```python
from build123d import *

# Parameters (mm, degrees)
EXTRUDE_START          = -12.5
EXTRUDE_1_DEPTH        = 25
EXTRUDE_ROTATE_1_ANGLE = 8
EXTRUDE_START_2        = -8.5
EXTRUDE_SKETCH_2_W     = 410
EXTRUDE_SKETCH_2_H     = 310
EXTRUDE_2_DEPTH        = 3
EXTRUDE_ROTATE_2_ANGLE = 8
EXTRUDE_START_3        = -30.5
EXTRUDE_SKETCH_3_W     = 80
EXTRUDE_SKETCH_3_H     = 80
EXTRUDE_3_DEPTH        = 22
EXTRUDE_ROTATE_3_ANGLE = 8


with BuildPart() as part:
    # Extrude sketch 1 → Extrude 1 (new body)
    with BuildSketch(Plane.XY.offset(EXTRUDE_START)):
        with BuildLine():
            Line((219, 175), (-219, 175))
            ThreePointArc((-219, 175), (-223.242640687, 173.242640687), (-225, 169))
            Line((-225, 169), (-225, -169))
            ThreePointArc((-225, -169), (-223.242640687, -173.242640687), (-219, -175))
            Line((-219, -175), (219, -175))
            ThreePointArc((219, -175), (223.242640687, -173.242640687), (225, -169))
            Line((225, -169), (225, 169))
            ThreePointArc((225, 169), (223.242640687, 173.242640687), (219, 175))
        make_face()
        with BuildLine():
            Line((203, 155), (-203, 155))
            ThreePointArc((-203, 155), (-204.414213562, 154.414213562), (-205, 153))
            Line((-205, 153), (-205, -153))
            ThreePointArc((-205, -153), (-204.414213562, -154.414213562), (-203, -155))
            Line((-203, -155), (203, -155))
            ThreePointArc((203, -155), (204.414213562, -154.414213562), (205, -153))
            Line((205, -153), (205, 153))
            ThreePointArc((205, 153), (204.414213562, 154.414213562), (203, 155))
        make_face(mode=Mode.SUBTRACT)
    extrude(amount=EXTRUDE_1_DEPTH)


with BuildPart() as part_1:
    # Extrude rotate 1: moved
    add(part.part.rotate(Axis((0, 0, 0), (0, 1, 0)), EXTRUDE_ROTATE_1_ANGLE))


with BuildPart() as part_2:
    # Extrude place 1: moved
    add(part_1.part.moved(Location((588.929348295, 0, 623.692298575))))


with BuildPart() as body_2:
    # Extrude sketch 2 → Extrude 2 (new body)
    with BuildSketch(Plane.XY.offset(EXTRUDE_START_2)):
        Rectangle(EXTRUDE_SKETCH_2_W, EXTRUDE_SKETCH_2_H)
    extrude(amount=EXTRUDE_2_DEPTH)


with BuildPart() as body_2_1:
    # Extrude rotate 2: moved
    add(body_2.part.rotate(Axis((0, 0, 0), (0, 1, 0)), EXTRUDE_ROTATE_2_ANGLE))


with BuildPart() as body_2_2:
    # Extrude place 2: moved
    add(body_2_1.part.moved(Location((588.929348295, 0, 623.692298575))))


with BuildPart() as body_3:
    # Extrude sketch 3 → Extrude 3 (new body)
    with BuildSketch(Plane.XY.offset(EXTRUDE_START_3)):
        with Locations((100, 0)):
            Rectangle(EXTRUDE_SKETCH_3_W, EXTRUDE_SKETCH_3_H)
    extrude(amount=EXTRUDE_3_DEPTH)


with BuildPart() as body_3_1:
    # Extrude rotate 3: moved
    add(body_3.part.rotate(Axis((0, 0, 0), (0, 1, 0)), EXTRUDE_ROTATE_3_ANGLE))


with BuildPart() as body_3_2:
    # Extrude place 3: moved
    add(body_3_1.part.moved(Location((588.929348295, 0, 623.692298575))))


with BuildPart() as part_3:
    add(part_2.part)

    # Combine (weld / assembly of features): union body 3, body 2
    add(body_3_2.part)
    add(body_2_2.part)


solid = part_3.part
```
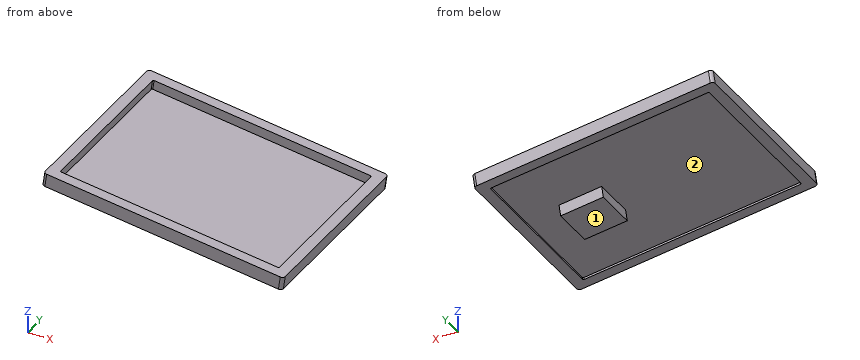
Part model, mm, in its own coordinate system. Face numbers are marked on the shaded views. Round coordinates to 2 decimals unless told otherwise and drop trailing zeros. Loops run counter-clockwise (first coordinate to the right, second up) from the corner with the lowest first, then second, coordinate; pieces in that order, holes last.
1. Slice it at C-C (x = 527). Give the cut face in (y, z).
Solutions:
outline: (-175, 619.77) - (-155, 619.77) - (-155, 623.81) - (155, 623.81) - (155, 619.77) - (175, 619.77) - (175, 645.02) - (155, 645.02) - (155, 626.84) - (-155, 626.84) - (-155, 645.02) - (-175, 645.02) - close
2. Slice it at A-A (y = 8). Give the cut face in (x, z), and give its area (3 significant figures).
Solutions:
outline: (364.38, 642.63) - (384.18, 639.84) - (384.74, 643.81) - (647.16, 606.92) - (644.1, 585.14) - (723.32, 574) - (726.38, 595.79) - (790.75, 586.74) - (790.19, 582.78) - (810, 580) - (813.48, 604.76) - (793.67, 607.54) - (791.17, 589.72) - (385.16, 646.78) - (387.66, 664.6) - (367.86, 667.38) - close
area: 3,990 mm2
3. Two-plate mould, pull along Y, no slides. Class the marked faces 1 and 2: pulls with the +Y half, pulls with the -Y half, needs draft (parallel to the pull), parting line crosses it, or undercut.
Solutions:
face 1: needs draft
face 2: undercut
4. Slice it at B-B (z = 623). Give the cut face in (x, y), and give its area (3 significant figures).
Solutions:
outline: (504.04, -175) - (683.67, -175) - (683.67, -155) - (554.34, -155) - (554.34, 155) - (683.67, 155) - (683.67, 175) - (504.04, 175) - (504.04, 155) - (532.78, 155) - (532.78, -155) - (504.04, -155) - close
area: 13,900 mm2
5. Slice it at D-D (x = 689). Give the cut face in (y, z), and give its area (3 significant figures).
Solutions:
outline: (-175, 597.01) - (-155, 597.01) - (-155, 601.04) - (-40, 601.04) - (-40, 578.83) - (40, 578.83) - (40, 601.04) - (155, 601.04) - (155, 597.01) - (175, 597.01) - (175, 622.25) - (155, 622.25) - (155, 604.07) - (-155, 604.07) - (-155, 622.25) - (-175, 622.25) - close
area: 3,730 mm2
6. Drill centre lines: line 1 along Y through (x, z) = (595, 621.5); line 2 along Z through (x, y) = (413, -25); line 3 along Z through (x, y) = (674.5, 103.5). Where is each one in solid material? Low to high.
Solutions:
line 1: y = -175 to -155, 155 to 175
line 2: z = 639.83 to 642.86
line 3: z = 603.08 to 606.11
7. Flat gauge pins, fed straight in: pin 1 (6 mm diameter, centred on x = 597, y = -23, fed in from +Z); pin 2 (16.5 mm diameter, centred on x = 672, z = 597, fed in from +Y); pin 3 (1.5 mm diameter, centred on x = 516, y = 99, fed in from -Z); pin 4 (5 mm diameter, centred on x = 532.5, y = 55, fed in from +Z). Where does each tip first touch, or does it go through?
Solutions:
pin 1: stops at z = 617.43
pin 2: stops at y = 175
pin 3: stops at z = 625.25
pin 4: stops at z = 626.42
